Job drawing, mm, ordinate dimensions from the low corner. One solid piece. Give positions to 0.01 mm unless a question says otherwise; leave off trailing zeros. Loops run counter-clockwise (first coordinate to the right, second up) from the corner with the lowest first, then second, coordinate; pieces in that order, holes last. Notation, with made-up numbers: M 67,22.5 L 89,22.5 A10 cw 89,28.5 Z; hole C -6.5,37.25 d4. An arc over 180 degrees is marked long. Put each result on its own line as item: value.
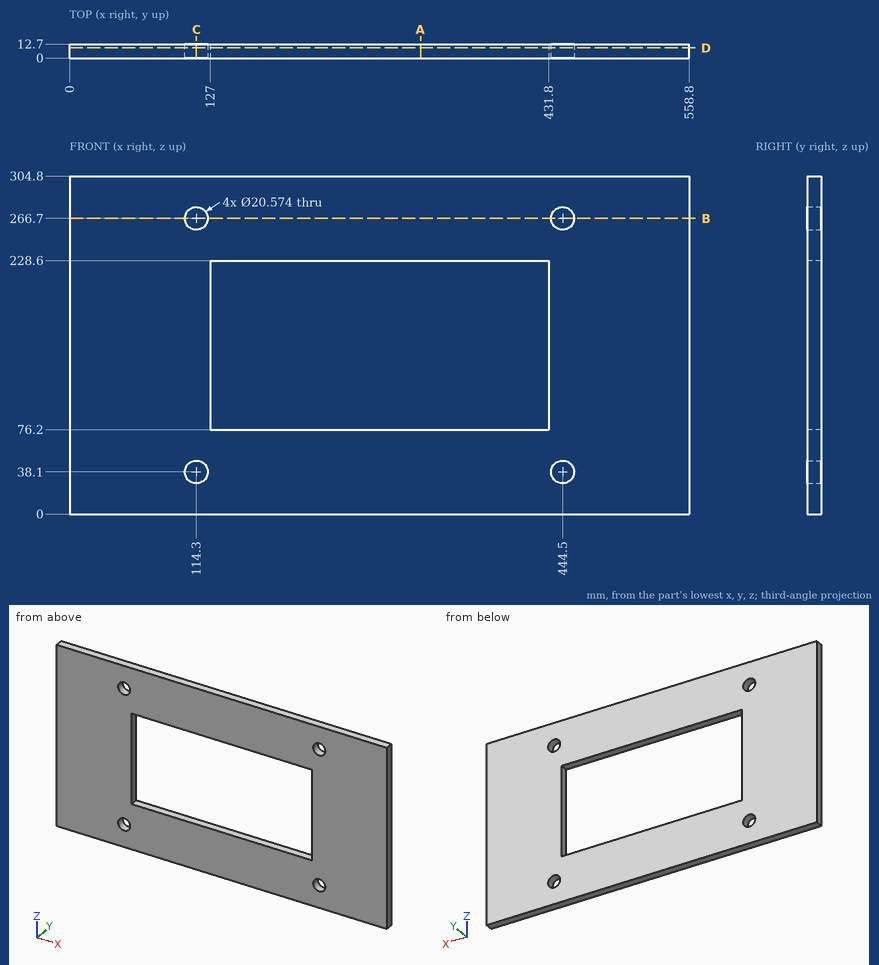
Q1. Slice it at D-D (y = 9.25). List the corners of the cut face in (x, z), and give its area (3 significant figures).
Here are the results:
outline: M 0,0 L 558.8,0 L 558.8,304.8 L 0,304.8 Z; hole C 114.3,38.1 d20.57; hole C 114.3,266.7 d20.57; hole M 127,76.2 L 431.8,76.2 L 431.8,228.6 L 127,228.6 Z; hole C 444.5,38.1 d20.57; hole C 444.5,266.7 d20.57
area: 123,000 mm²
Q2. Drop a flat-ended pin along its axis: pin 1 Ø16.5 at (x, z) = (114.3, 266.7) entering from +Y. Give the stop position or say it passes through.
Here are the results:
pin 1: through
Q3. Slice it at B-B (z = 266.7). List the corners of the cut face in (x, y).
Here are the results:
outline: M 0,0 L 104.01,0 L 104.01,12.7 L 0,12.7 Z; M 124.59,0 L 434.21,0 L 434.21,12.7 L 124.59,12.7 Z; M 454.79,0 L 558.8,0 L 558.8,12.7 L 454.79,12.7 Z
Q4. Slice it at C-C (x = 114.3). List the corners of the cut face in (y, z), and give its area (3 significant figures).
Here are the results:
outline: M 0,0 L 12.7,0 L 12.7,27.81 L 0,27.81 Z; M 0,48.39 L 12.7,48.39 L 12.7,256.41 L 0,256.41 Z; M 0,276.99 L 12.7,276.99 L 12.7,304.8 L 0,304.8 Z
area: 3,350 mm²
Q5. Slice it at A-A (x = 316.5). List the corners of the cut face in (y, z).
Here are the results:
outline: M 0,0 L 12.7,0 L 12.7,76.2 L 0,76.2 Z; M 0,228.6 L 12.7,228.6 L 12.7,304.8 L 0,304.8 Z
Q6. Probe line 1 (X direction, y = 6, z = 38.1); line 2 (Z direction, x = 444.5, y = 2.5); line 3 (X direction, y = 10.5, z = 265.5). List the from-to ranges inside material, lowest first. Write a range as from..to.
Here are the results:
line 1: 0..104.01, 124.59..434.21, 454.79..558.8
line 2: 0..27.81, 48.39..256.41, 276.99..304.8
line 3: 0..104.08, 124.52..434.28, 454.72..558.8
